```python
from build123d import *

# Parameters (mm, degrees)
EXTRUDE_1_DEPTH      = 3
EXTRUDE_1_DEPTH_BACK = 3


with BuildPart() as part:
    # Sketch 1 → Extrude 1 (new body, two sides)
    with BuildSketch(Plane.XY) as extrude_1_sk:
        with BuildLine():
            Line((-5.483999587, -12.650498258), (38.980167841, -31.925745039))
            ThreePointArc((38.980167841, -31.925745039), (87.6164675, 0), (38.980167841, 31.925745039))
            Line((38.980167841, 31.925745039), (-5.483999587, 12.650498258))
            ThreePointArc((-5.483999587, 12.650498258), (-13.788015, 0), (-5.483999587, -12.650498258))
        make_face()
        with BuildLine():
            Line((-5.165810227, -11.916498577), (39.298357201, -31.191745358))
            ThreePointArc((39.298357201, -31.191745358), (86.8164675, 0), (39.298357201, 31.191745358))
            Line((39.298357201, 31.191745358), (-5.165810227, 11.916498577))
            ThreePointArc((-5.165810227, 11.916498577), (-12.988015, 0), (-5.165810227, -11.916498577))
        make_face(mode=Mode.SUBTRACT)
    extrude(amount=EXTRUDE_1_DEPTH)
    extrude(extrude_1_sk.sketch, amount=-EXTRUDE_1_DEPTH_BACK)


solid = part.part
```
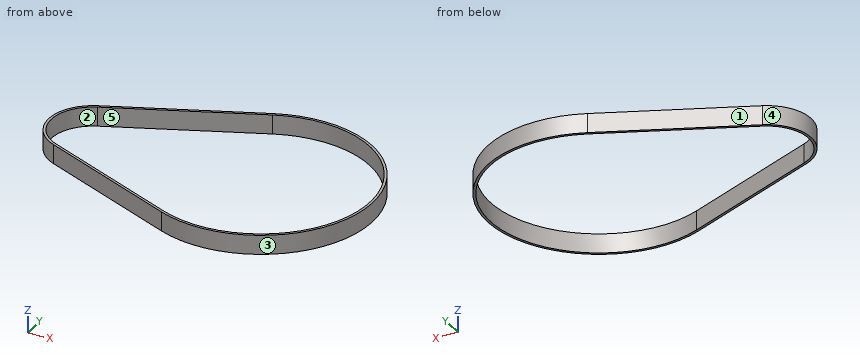
Source: CAD feature listing. Evaluate the final solid. Frame: model axes, mm. Face numbers are marked on the shaded views. A direction names the side the tool comes from. Coordinates: 2 decimals unless noted, no trailing zeros. Loops run counter-clockwise (first coordinate to the right, second up) from the corner with the lowest first, then second, coordinate; pieces in that order, holes last. Notation, with made-up numbers: M 83.25,-7 L 89.25,-7 A23 ccw 89.25,15 Z; hole C -29,2.5 d6. An arc over 180 degrees is marked long. Put each result on its own line as item: value. Start each with the question number.
1) Contact query for flat-ended pins moving along their axis: pin 1 Ø5 at (x, y) = (24.5, -22) entering from +Z; pin 2 Ø1.5 at (x, z) = (-3.5, -2) entering from +Y. Output: stop coordinate, or through.
2) Cut plane A-A on z = 1.35. Return the cut outline in (x, y).
3) Pull-direction query (X, two-part tool) for the marked faces 1, 2 and 3; classes: pulls with the +X half, pulls with the -X half, needs draft (parallel to the pull), parting line crosses it, or undercut.
4) Cut plane B-B on y = 0. Return the cut outline in (x, z).
5) Cut plane C-C on x = 52.82. Return the cut outline in (y, z).
6) Reachability of the marked faces 4 and 5 from +Z, -Z, +X, -X, +Y, -Y: full face, straight path, thin tool, end or side. Return the list, or none.
7) Ray query, L1, parallel to Y at x = 52.82, z = 0.35; L2, parallel to X at y = 15.5, z = 2.6; L3, parallel to X at y = 2, z = 0.85. Return the intervals inside material, ascending. Write a range as from..to.
The answers:
1. pin 1: passes through
1. pin 2: stops at y = 13.84
2. outline: M -5.48,-12.65 L 38.98,-31.93 A34.8 ccw long 38.98,31.93 L -5.48,12.65 A13.79 ccw Z; hole M -5.17,-11.92 L 39.3,-31.19 A34 ccw long 39.3,31.19 L -5.17,11.92 A12.99 ccw Z
3. face 1: pulls with the -X half
3. face 2: undercut
3. face 3: parting line crosses it
4. outline: M -13.79,-3 L -12.99,-3 L -12.99,3 L -13.79,3 Z; M 86.82,-3 L 87.62,-3 L 87.62,3 L 86.82,3 Z
5. outline: M -34.8,-3 L -34,-3 L -34,3 L -34.8,3 Z; M 34,-3 L 34.8,-3 L 34.8,3 L 34,3 Z
6. face 4: +Z, -Z, -X
6. face 5: +Z, -Z
7. L1: y = -34.8..-34, 34..34.8
7. L2: x = 1.09..3.1, 83.08..83.97
7. L3: x = -13.64..-12.83, 86.76..87.56
